from build123d import *

# Parameters (mm, degrees)
SKETCH2_R           = 30
BOSS_EXTRUDE1_DEPTH = 125
CUT_EXTRUDE1_START  = -50
CUT_EXTRUDE1_DEPTH  = 50


with BuildPart() as part:
    # Sketch2 → Boss-Extrude1 (new, symmetric)
    with BuildSketch(Plane(origin=(0, 0, 0), x_dir=(1, 0, 0), z_dir=(0, 1, 0))):
        with Locations(Location((0, 0, 0), (0, 0, 270))):
            Circle(SKETCH2_R)
    extrude(amount=BOSS_EXTRUDE1_DEPTH, both=True)

    # Sketch3 → Cut-Extrude1 (cut)
    with BuildSketch(Plane.XZ.offset(125).offset(CUT_EXTRUDE1_START)):
        with BuildLine():
            ThreePointArc((-8.095335695, 28.887117197), (0, 30), (8.095335695, 28.887117197))
            Line((8.095335695, 28.887117197), (8.095335695, 34.42))
            Line((8.095335695, 34.42), (-8.095335695, 34.42))
            Line((-8.095335695, 34.42), (-8.095335695, 28.887117197))
        make_face()
        with BuildLine():
            Line((-8.095335695, 27.42), (8.095335695, 27.42))
            Line((8.095335695, 27.42), (8.095335695, 28.887117197))
            ThreePointArc((8.095335695, 28.887117197), (0, 30), (-8.095335695, 28.887117197))
            Line((-8.095335695, 28.887117197), (-8.095335695, 27.42))
        make_face()
    extrude(amount=CUT_EXTRUDE1_DEPTH, mode=Mode.SUBTRACT)


solid = part.part
The listing builds one solid part. Answer for the finished solid, in the listing's coordinates (mm). Round coordinates to 2 decimals unless told otherwise and drop trailing zeros. Write each loop counter-clockwise with the first axis right and the second up, starting at its lowest first coordinate (ties: lowest second). Pieces come first, ordered by that corner, then holes. Notation, with made-up numbers: (-23.5, 39) - (-19.5, 39) arc R34 cw to (-19.5, 73) - close; hole circle Ø1 at (-6.5, 25.5). An arc over 180 degrees is marked (long way). Use a Markdown table: item, result. Add a question column.
1. The part is cut by section B-B (x = 13.5). Write down the section's boundary in (y, z), and give its area (3 significant figures).
2. Consider line 1 (X direction, y = 5.5, z = 0); line 2 (Z direction, x = -1.5, y = 0); line 3 (X direction, y = -32, z = 4). Determine where each line is inside the solid, lowest interval first.
3. Flat-ended cylindrical pins translate along their axes: P1, Ø8, axis at y = -19, z = 19, coming from the -X side; P2, Ø12, axis at x = -17.5, y = 63, coming from the -Z side; P3, Ø8, axis at x = -9, y = -85, coming from the -Z side. Find the tip coordinate at first contact, or state that the pin passes through.
4. For a pull along X with two mould halves and no side action, classify faces 1 (the face through (0, -125, -1)), 2 (the face through (1.32, 1.75, -29.97)), 3 (the face through (0, -100, 27.42)) as +X half, -X half, draft (parallel to the pull), parting line (faces both ways), or undercut.
5. The part is cut by section A-A (y = -97.5). Write down the section's boundary in (x, z), and give its area (3 significant figures).
6. The part is cut by section C-C (y = -47.5). Write down the section's boundary in (x, z).
Reported:
| question | item | result |
|---|---|---|
| 1 | outline | (-125, -26.79) - (125, -26.79) - (125, 26.79) - (-125, 26.79) - close |
| 1 | area | 13,400 mm^2 |
| 2 | line 1 | -30 to 30 |
| 2 | line 2 | -29.96 to 29.96 |
| 2 | line 3 | -29.73 to 29.73 |
| 3 | P1 | x = -25.98 |
| 3 | P2 | z = -27.71 |
| 3 | P3 | z = -29.58 |
| 4 | face 1 | draft |
| 4 | face 2 | parting line |
| 4 | face 3 | undercut |
| 5 | outline | (-8.1, 27.42) - (-8.1, 28.89) arc R30 ccw (long way) to (8.1, 28.89) - (8.1, 27.42) - close |
| 5 | area | 2,790 mm^2 |
| 6 | outline | circle Ø60 at (0, 0) |
